from build123d import *

# Parameters (mm, degrees)
EXTRUDE_1_DEPTH      = 3
EXTRUDE_2_DEPTH      = 100
SKETCH_3_W           = 26.5
SKETCH_3_H           = 26.50000000000003
SKETCH_3_W_2         = 26.500000000000004
SKETCH_3_H_2         = 26.5
EXTRUDE_3_DEPTH      = 75
FILLET_2_R           = 20
FILLET_3_R           = 20
FILLET_6_R           = 10
EXTRUDE_7_DEPTH      = 20
SKETCH_14_W          = 22.50000000000002
SKETCH_14_H          = 65
EXTRUDE_8_DEPTH      = 20
SKETCH_15_W          = 102.75181222829023
SKETCH_15_H          = 15
CUT_EXTRUDE_6_DEPTH  = 2.99999999999999
FILLET_7_R           = 90
FILLET_8_R           = 30
SKETCH_17_W          = 62.00000000000001
SKETCH_17_H          = 15
CUT_EXTRUDE_8_DEPTH  = 2.99999999999999
FILLET_9_R           = 5
FILLET_11_R          = 20
FILLET_12_R          = 20
FILLET_13_R          = 10
CUT_EXTRUDE_9_DEPTH  = 300
SKETCH_19_R          = 1.0000000000000018
SKETCH_19_R_2        = 1
SKETCH_19_R_3        = 1.0000000000000033
CUT_EXTRUDE_12_DEPTH = 18
SKETCH_19_4_W        = 2
SKETCH_19_4_H        = 25
SKETCH_19_4_W_2      = 2.0000000000000018
CUT_EXTRUDE_13_DEPTH = 20
FILLET_15_R          = 1


# Some blends are built 0.0001 mm under size
with BuildPart() as part:
    # Эскиз1 → Бобышка-Вытянуть1 (new body)
    with BuildSketch(Plane(origin=(0, 0, 0), x_dir=(1, 0, 0), z_dir=(0, 1, 0))):
        Polygon((0, 0), (-130, -1.837e-14), (-130, 129.99999999999997), (0, 130), align=None)
    extrude(amount=EXTRUDE_1_DEPTH)

    # Эскиз2 → Бобышка-Вытянуть2 (add)
    with BuildSketch(Plane(origin=(0, 3, 0), x_dir=(1, 0, 0), z_dir=(0, 1, 0))):
        Polygon((-130, 129.99999999999997), (-55.00000000000002, 130.0000000000001), (-55.00000000000002, 55.0000000000001), (-130.00000000000003, 55.0000000000001), align=None)
        Polygon((-127, 126.99999999999997), (-58.00000000000002, 127.00000000000009), (-58.000000000000014, 58.0000000000001), (-127.00000000000003, 58.00000000000009), align=None, mode=Mode.SUBTRACT)
    extrude(amount=EXTRUDE_2_DEPTH)

    # Эскиз3 → Бобышка-Вытянуть3 (add)
    # profile 1 of 2: a face of its own
    with BuildSketch(Plane(origin=(0, 3, 0), x_dir=(1, 0, 0), z_dir=(0, 1, 0))):
        Polygon((-22.50000000000002, 130), (-55.00000000000002, 130), (-55.00000000000002, 97.5), (-22.500000000000014, 97.5), align=None)
        with Locations((-38.75000000000002, 113.75)):
            Rectangle(SKETCH_3_W, SKETCH_3_H, mode=Mode.SUBTRACT)
    # profile 2 of 2: a face of its own
    with BuildSketch(Plane(origin=(0, 3, 0), x_dir=(1, 0, 0), z_dir=(0, 1, 0))):
        Polygon((-22.500000000000014, 97.5), (-55.00000000000002, 97.5), (-55.00000000000002, 65), (-22.5, 65), align=None)
        with Locations((-38.750000000000014, 81.25)):
            Rectangle(SKETCH_3_W_2, SKETCH_3_H_2, mode=Mode.SUBTRACT)
    extrude(amount=EXTRUDE_3_DEPTH)

    # Скругление2
    fillet_2_edges = [part.edges().sort_by_distance(p)[0] for p in [
        (-127, 53, -126.99999999999997),
        (-130, 51.5, -129.99999999999997),
    ]]
    fillet(fillet_2_edges, radius=FILLET_2_R)

    # Скругление3
    fillet_3_edges = [part.edges().sort_by_distance(p)[0] for p in [
        (-58.000000000000014, 53, -58.0000000000001),
        (-55.00000000000002, 53, -55.0000000000001),
        (-58.00000000000002, 53, -127.00000000000009),
        (-55.00000000000002, 90.5, -130.0000000000001),
    ]]
    fillet(fillet_3_edges, radius=FILLET_3_R)

    # Скругление6
    fillet_6_edges = [part.edges().sort_by_distance(p)[0] for p in [
        (-57.6794919243113, 40.5, -65),
        (-52.000000000000014, 40.5, -94.50000000000001),
        (-25.500000000000014, 40.5, -94.50000000000001),
        (-25.500000000000014, 40.5, -68),
        (-52.00000000000003, 40.5, -127),
        (-25.50000000000002, 40.5, -127),
        (-25.50000000000002, 40.5, -100.49999999999999),
        (-52.00000000000003, 40.5, -100.49999999999999),
        (-52.000000000000014, 40.5, -68),
    ]]
    fillet(fillet_6_edges, radius=FILLET_6_R)

    # Эскиз4 → Бобышка-Вытянуть7 (add)
    with BuildSketch(Plane(origin=(0, 3, 0), x_dir=(1, 0, 0), z_dir=(0, 1, 0))):
        Polygon((-3, 65), (-3, 2.999999999999999), (0, 2.999999999999982), (0, 65), align=None)
        Polygon((-3, 2.999999999999982), (-126.99999999999997, 2.999999999999982), (-126.99999999999997, -2.132e-14), (0, -1.721e-14), (0, 2.999999999999982), align=None)
        Polygon((-127, 55.0000000000001), (-130, 55.0000000000001), (-130, -1.421e-14), (-126.99999999999997, -1.837e-14), (-126.99999999999997, 2.9999999999999787), align=None)
    extrude(amount=EXTRUDE_7_DEPTH)

    # Эскиз14 → Бобышка-Вытянуть8 (add)
    with BuildSketch(Plane(origin=(0, 3, 0), x_dir=(1, 0, 0), z_dir=(0, 1, 0))):
        with Locations((-11.25000000000001, 97.5)):
            Rectangle(SKETCH_14_W, SKETCH_14_H)
    extrude(amount=EXTRUDE_8_DEPTH)

    # Эскиз15 → Вырез-Вытянуть6 (cut)
    with BuildSketch(Plane.XY):
        with Locations((-51.37590611414512, 15.5)):
            Rectangle(SKETCH_15_W, SKETCH_15_H)
    extrude(amount=-CUT_EXTRUDE_6_DEPTH, mode=Mode.SUBTRACT)

    # Скругление7
    # the kernel refuses this fillet: 90 mm, written as the material it adds along each edge
    with BuildSketch(Plane(origin=(-102.75181222829023, 8, 0), x_dir=(-9.5e-16, 1, 0), z_dir=(0, 0, -1))) as fillet_7_piece_1:
        with BuildLine():
            CenterArc((89.99999999999996, 49.74937185533107), FILLET_7_R, 180.00000000000006, 33.55730976192069)
            Line((-4.713e-14, 49.749371855330985), (-1.800000000000047, 49.749371855330985))
            Line((-1.800000000000047, 49.749371855330985), (-1.7999999999999998, -1.71e-15))
            Line((-1.7999999999999998, -1.71e-15), (1.71e-15, -1.7999999999999972))
            ThreePointArc((1.71e-15, -1.7999999999999972), (7.499999999999995, -1.79999999999999), (13.499999999999988, -0.9949874371066173))
            Line((13.499999999999988, -0.9949874371066173), (14.999999999999986, 0))
        make_face()
    extrude(amount=2.99999999999999)

    # Скругление8
    fillet_8_edges = [part.edges().sort_by_distance(p)[0] for p in [
        (-102.75181222829023, 23, -1.499999999999995),
    ]]
    fillet(fillet_8_edges, radius=FILLET_8_R)

    # Эскиз17 → Вырез-Вытянуть8 (cut)
    with BuildSketch(Plane(origin=(0, 0, 0), x_dir=(0, 0, -1), z_dir=(1, 0, 0))):
        with Locations((33.99999999999999, 15.5)):
            Rectangle(SKETCH_17_W, SKETCH_17_H)
    extrude(amount=-CUT_EXTRUDE_8_DEPTH, mode=Mode.SUBTRACT)

    # Скругление9
    fillet_9_edges = [part.edges().sort_by_distance(p)[0] for p in [
        (-126.99999999999997, 13, -2.9999999999999805),
        (-3, 5.5, -2.9999999999999902),
        (0, 4, 2.99e-15),
        (-130, 11.5, 1.704e-14),
        (0, 11.5, -130),
    ]]
    fillet(fillet_9_edges, radius=FILLET_9_R)

    # Скругление11
    fillet_11_edges = [part.edges().sort_by_distance(p)[0] for p in [
        (-127.00000000000003, 53, -58.00000000000009),
    ]]
    fillet(fillet_11_edges, radius=FILLET_11_R)

    # Скругление12
    fillet_12_edges = [part.edges().sort_by_distance(p)[0] for p in [
        (-130.00000000000003, 63, -55.0000000000001),
    ]]
    fillet(fillet_12_edges, radius=FILLET_12_R)

    # Скругление13
    fillet_13_edges = [part.edges().sort_by_distance(p)[0] for p in [
        (-22.5, 50.5, -65),
        (-22.50000000000002, 50.5, -130),
    ]]
    fillet(fillet_13_edges, radius=FILLET_13_R)

    # Эскиз18 → Вырез-Вытянуть9 (cut)
    with BuildSketch(Plane.XY.offset(-65)):
        Polygon((-22.50000000000001, 22.999999999999993), (0, 18), (0, 23), align=None)
    extrude(amount=-CUT_EXTRUDE_9_DEPTH, mode=Mode.SUBTRACT)

    # Эскиз19 → Вырез-Вытянуть12 (cut)
    with BuildSketch(Plane(origin=(3.811764705882347, 17.15294117647059, 0), x_dir=(0.9761870601839528, -0.2169304578186562, 0), z_dir=(0.2169304578186562, 0.9761870601839528, 0))):
        with Locations(Location((-9.666963526543862, 102.5, 0), (0, 0, 180))):
            Circle(SKETCH_19_R)
        with Locations(Location((-9.666963526543864, 107.5, 0), (0, 0, 180))):
            Circle(SKETCH_19_R_2)
        with Locations(Location((-9.666963526543864, 112.49999999999999, 0), (0, 0, 180))):
            Circle(SKETCH_19_R_2)
        with Locations(Location((-9.666963526543865, 117.49999999999999, 0), (0, 0, 180))):
            Circle(SKETCH_19_R)
        with Locations(Location((-9.666963526543862, 97.5, 0), (0, 0, 180))):
            Circle(SKETCH_19_R)
        with Locations(Location((-9.666963526543793, 92.50000000000001, 0), (0, 0, 180))):
            Circle(SKETCH_19_R)
        with Locations(Location((-9.666963526543721, 87.50000000000001, 0), (0, 0, 180))):
            Circle(SKETCH_19_R_2)
        with Locations(Location((-9.666963526543652, 82.50000000000001, 0), (0, 0, 180))):
            Circle(SKETCH_19_R_3)
        with Locations(Location((-9.66696352654358, 77.50000000000003, 0), (0, 0, 180))):
            Circle(SKETCH_19_R)
    extrude(amount=-CUT_EXTRUDE_12_DEPTH, mode=Mode.SUBTRACT)

    # Эскиз19<4> → Вырез-Вытянуть13 (cut)
    with BuildSketch(Plane(origin=(3.811764705882347, 17.15294117647059, 0), x_dir=(0.9761870601839528, -0.2169304578186562, 0), z_dir=(0.2169304578186562, 0.9761870601839528, 0))):
        Polygon((-22.191394098159968, 125.00000000000003), (-22.191394098159964, 100), (-20.191394098159968, 100), (-20.19139409815997, 125.00000000000003), align=None)
        Polygon((-20.191394098159975, 95.00000000000003), (-20.19139409815997, 70), (-22.191394098159968, 70), (-22.19139409815997, 95.00000000000003), align=None)
        with Locations((-15.429178812351914, 112.50000000000001)):
            Rectangle(SKETCH_19_4_W, SKETCH_19_4_H)
        with Locations((-15.429178812351918, 82.5)):
            Rectangle(SKETCH_19_4_W_2, SKETCH_19_4_H)
    extrude(amount=-CUT_EXTRUDE_13_DEPTH, mode=Mode.SUBTRACT)

    # Скругление15
    fillet_15_edges = [part.edges().sort_by_distance(p)[0] for p in [
        (-14.395491638370515, 10.95505985597913, -100),
        (-20.020491638370512, 12.205059855979126, -100),
        (-14.395491638370515, 10.95505985597913, -125),
        (-20.020491638370515, 12.20505985597913, -125.00000000000003),
        (-18.068117518002612, 11.771198940341815, -100),
        (-12.44311751800261, 10.521198940341815, -100),
        (-12.44311751800261, 10.521198940341815, -125),
        (-18.068117518002612, 11.771198940341815, -125.00000000000003),
        (-12.443117518002612, 10.521198940341815, -95),
        (-18.068117518002616, 11.771198940341819, -95.00000000000003),
        (-14.395491638370519, 10.95505985597913, -95),
        (-20.02049163837052, 12.20505985597913, -95.00000000000003),
        (-12.443117518002612, 10.521198940341815, -70),
        (-18.068117518002612, 11.771198940341815, -70),
        (-14.395491638370519, 10.95505985597913, -70),
        (-20.020491638370515, 12.20505985597913, -70),
    ]]
    fillet(fillet_15_edges, radius=FILLET_15_R - 0.0001)  # a hair under: the kernel refuses the full size


solid = part.part
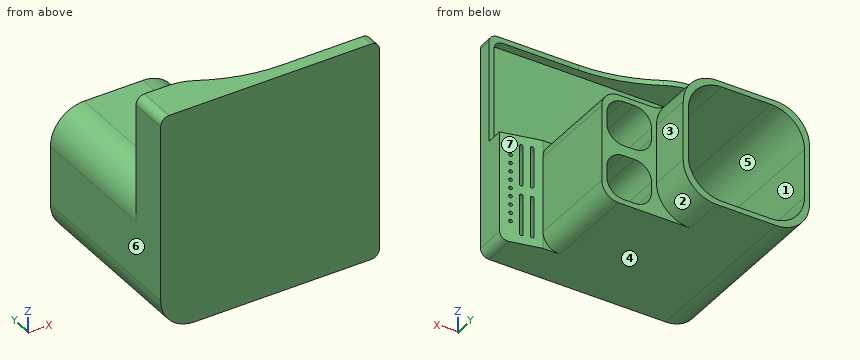
Input: part model. Units: mm. Frame: model coordinates. Face numbers are marked on the shaded views. A direction names the side the tool comes from. Give positions to 0.01 mm unless a question says otherwise; leave off trailing zeros. Write each loop counter-clockwise with the first axis right and the second up, starting at its lowest first coordinate (ties: lowest second). Pieces come first, ordered by that corner, then holes. Notation, with made-up numbers: (70, 44) -> (104, 44) arc R29 cw to (104, 65) -> close; hole circle Ø1 at (-32, 25). An arc over 180 degrees is marked (long way). Use one line per item in the form item = value. Start each with the question number.
1) Section query B-B on z = -44. Return the cut outline in (x, y).
2) Section query A-A on y = 94.5. Return the cut outline in (x, z).
3) Draft query along X for the marked faces 4, 5, 6 and 7. Return one class per face: pulls with the +X half, pulls with the -X half, needs draft (parallel to the pull), parting line crosses it, or undercut.
4) Section query D-D on y = 54. Count the separate pieces of the cut face and the enclosed holes in it, then the cut area to 3 significant figures.
5) Ray query, probe 1 along Z at (x, y) = (-42, 7); probe 2 along Z at (x, y) = (-41.5, 15.5); probe 3 along Z at (x, y) = (-15, 6.5). Return the intervals inside material, ascending. Write a range as from..to.
6) Set-up query: the marked faces 1, 2 and 3. Return all of +Z, -Z, +X, -X, +Y, -Y with unobstructed straight access to the full face (end or side cutting, diameter ignored); none if empty.
7) Pin query (flat end, axial travel): pin 1 (10 mm diameter, centred on y = 17.5, z = -22, fed in from +X); pin 2 (5 mm diameter, centred on x = -59, y = 11, fed in from +Z); pin 3 (5 mm diameter, centred on x = -26.5, z = -126, fed in from +Y). Return the tip coordinate at first contact, or that it passes through.
8) Section query C-C on x = -47.5. Return the cut outline in (y, z), then the cut area to 3 significant figures.
Outcome:
q1.outline = (-130, 0) -> (0, 0) -> (0, 8) -> (-3, 8) -> (-3, 3) -> (-127, 3) -> (-127, 23) -> (-130, 23) -> close
q2.outline = (-130, -110) arc R20 ccw to (-110, -130) -> (-75, -130) arc R20 ccw to (-55, -110) -> (-55, -75) arc R20 ccw to (-75, -55) -> (-110, -55) arc R20 ccw to (-130, -75) -> close; hole (-127, -107) arc R20 ccw to (-107, -127) -> (-78, -127) arc R20 ccw to (-58, -107) -> (-58, -78) arc R20 ccw to (-78, -58) -> (-107, -58) arc R20 ccw to (-127, -78) -> close
q3.face_4 = needs draft
q3.face_5 = undercut
q3.face_6 = pulls with the -X half
q3.face_7 = pulls with the +X half
q4.separate_pieces = 1
q4.enclosed_holes = 3
q4.area = 1,800 mm^2
q5.probe_1 = -130..-127, -100.5..-94.5, -68..-65, -3..0
q5.probe_2 = -130..-127, -100.5..-94.5, -68..-65
q5.probe_3 = -130..-124.78, -100.22..-94.78, -70.22..-65, -3..0
q6.face_1 = +Y
q6.face_2 = -Z, +X, +Y
q6.face_3 = +Z, -Z, +X, +Y
q7.pin_1 = -127
q7.pin_2 = -60.24
q7.pin_3 = 78
q8.outline = (0, -130) -> (78, -130) -> (78, -125.35) -> (3, -125.35) -> (3, -102.15) -> (78, -102.15) -> (78, -92.85) -> (3, -92.85) -> (3, -69.65) -> (78, -69.65) -> (78, -65) -> (3, -65) -> (3, -3) -> (8, -3) -> (8, 0) -> (0, 0) -> close
q8.area = 1,800 mm^2
